from build123d import *

# Parameters (mm, degrees)
SKETCH1_W                    = 7.7
SKETCH1_H                    = 10
BASE_FLANGE1_DEPTH           = 3
EDGE_FLANGE1_STRIP_W         = 13.4732
EDGE_FLANGE1_STRIP_H         = 3
EDGE_FLANGE1_STRIP_CUT_DEPTH = 10
EDGE_FLANGE1_DEPTH           = 10
TAB1_START                   = -3
TAB1_OUTLINE_W               = 23
TAB1_OUTLINE_H               = 10
TAB1_DEPTH                   = 3
FILLET1_R                    = 0.6
FILLET2_R                    = 2
SKETCH15_R                   = 1.75
CUT_EXTRUDE1_DEPTH           = 22.318771072
EDGE_FLANGE2_START           = 2
EDGE_FLANGE2_DEPTH           = 10
EDGE_FLANGE2_2_DEPTH         = 10
CUT_EXTRUDE2_DEPTH           = 31.724582991
FILLET3_R                    = 2


# Read off the part's stored shape, not the designer's step: Tab1, Edge-Flange2
# Sheet-metal steps are written as plain solids
with BuildPart() as part:
    # Sketch1 → Base-Flange1 (new body)
    with BuildSketch(Plane(origin=(0, 0, 0), x_dir=(1, 0, 0), z_dir=(0, 1, 0))):
        with Locations((3.85, 0)):
            Rectangle(SKETCH1_W, SKETCH1_H)
    extrude(amount=-BASE_FLANGE1_DEPTH)

    # Edge-Flange1 strip (across the edge) → Edge-Flange1 strip cut (cut)
    with BuildSketch(Plane(origin=(7.7, 0, 5), x_dir=(-1, 0, 0), z_dir=(0, 0, -1))):
        with Locations((-6, -1.5)):
            Rectangle(EDGE_FLANGE1_STRIP_W, EDGE_FLANGE1_STRIP_H)
    extrude(amount=EDGE_FLANGE1_STRIP_CUT_DEPTH, mode=Mode.SUBTRACT)

    # Edge-Flange1 section (across the edge) → Edge-Flange1 (add)
    with BuildSketch(Plane(origin=(7.7, 0, 5), x_dir=(-1, 0, 0), z_dir=(0, 0, -1))):
        with BuildLine():
            Line((-3, 0.7366), (-3, 2))
            Line((-3, 2), (0, 2))
            Line((0, 2), (0, 0.7366))
            ThreePointArc((0, 0.7366), (0.215745145, 0.215745145), (0.7366, 0))
            Line((0.7366, 0), (0.7366, -3))
            ThreePointArc((0.7366, -3), (-1.905575199, -1.905575199), (-3, 0.7366))
        make_face()
    extrude(amount=EDGE_FLANGE1_DEPTH)

    # Tab1 outline → Tab1 (add)
    with BuildSketch(Plane(origin=(10.7, 0, 0), x_dir=(0, 0, -1), z_dir=(1, 0, 0)).offset(TAB1_START)):
        with Locations((2.5, 7)):
            Rectangle(TAB1_OUTLINE_W, TAB1_OUTLINE_H)
    extrude(amount=TAB1_DEPTH)

    # Fillet1
    fillet1_edges = [part.edges().sort_by_distance(p)[0] for p in [
        (9.2, 2, 5),
        (9.2, 2, -5),
    ]]
    fillet(fillet1_edges, radius=FILLET1_R)

    # Fillet2
    fillet2_edges = [part.edges().sort_by_distance(p)[0] for p in [
        (9.2, 12, -14),
        (9.2, 2, -14),
    ]]
    fillet(fillet2_edges, radius=FILLET2_R)

    # Sketch15 → Cut-Extrude1 (cut, through all)
    with BuildSketch(Plane(origin=(10.7, 0, 0), x_dir=(0, 0, -1), z_dir=(1, 0, 0))):
        with Locations(Location((9, 7, 0), (0, 0, 90))):
            Circle(SKETCH15_R)
    extrude(amount=-CUT_EXTRUDE1_DEPTH, mode=Mode.SUBTRACT)

    # Edge-Flange2 outline → Edge-Flange2 (cut)
    with BuildSketch(Plane(origin=(0, 0, 0), x_dir=(1, 0, 0), z_dir=(0, 1, 0)).offset(EDGE_FLANGE2_START)):
        with BuildLine():
            Line((10.7, -9), (10.7, -8.926677222))
            ThreePointArc((10.7, -8.926677222), (8.545704021, -7.630867001), (7.7, -5.2634))
            Line((7.7, -5.2634), (7.7, -9))
            Line((7.7, -9), (10.7, -9))
        make_face()
    extrude(amount=EDGE_FLANGE2_DEPTH, mode=Mode.SUBTRACT)

    # Edge-Flange2 2 outline → Edge-Flange2 2 (add)
    with BuildSketch(Plane(origin=(0, 0, 0), x_dir=(1, 0, 0), z_dir=(0, 1, 0)).offset(EDGE_FLANGE2_START)):
        with BuildLine():
            ThreePointArc((10.7, -8.926677222), (11.06647982, -8.981624121), (11.4366, -9))
            Line((11.4366, -9), (20, -9))
            Line((20, -9), (20, -6))
            Line((20, -6), (11.4366, -6))
            ThreePointArc((11.4366, -6), (10.915745145, -5.784254855), (10.7, -5.2634))
            Line((10.7, -5.2634), (10.7, -8.926677222))
        make_face()
    extrude(amount=EDGE_FLANGE2_2_DEPTH)

    # Sketch23 → Cut-Extrude2 (cut, through all)
    with BuildSketch(Plane(origin=(0, 0, 6), x_dir=(-1, 0, 0), z_dir=(0, 0, -1))):
        with BuildLine():
            Line((-15.75, 8.65), (-14.25, 8.65))
            ThreePointArc((-14.25, 8.65), (-12.6, 7), (-14.25, 5.35))
            Line((-14.25, 5.35), (-15.75, 5.35))
            ThreePointArc((-15.75, 5.35), (-17.4, 7), (-15.75, 8.65))
        make_face()
    extrude(amount=-CUT_EXTRUDE2_DEPTH, mode=Mode.SUBTRACT)

    # Fillet3
    fillet3_edges = [part.edges().sort_by_distance(p)[0] for p in [
        (20, 12, 7.5),
        (20, 2, 7.5),
    ]]
    fillet(fillet3_edges, radius=FILLET3_R)

    # Mirror1: part across plane


with BuildPart() as part_1:
    add(part.part)
    add(part.part.mirror(Plane(origin=(0, -3, -5), x_dir=(0, 0, 1), z_dir=(-1, 0, 0))))


solid = part_1.part
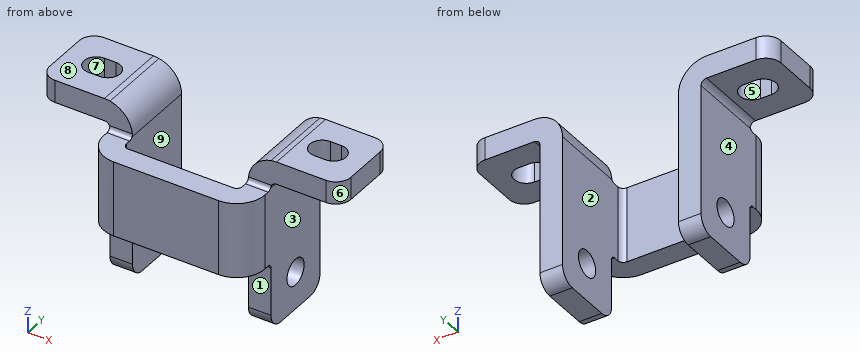
Could you check a few things on this model? Use its own coordinates, in mm. Face numbers are marked on the shaded views. A direction names the side the tool comes from. Coordinates: 2 decimals unless noted, no trailing zeros. Loops run counter-clockwise (first coordinate to the right, second up) from the corner with the lowest first, then second, coordinate; pieces in that order, holes last. Notation, with made-up numbers: (11.5, -35) -> (30.5, -35) arc R19 cw to (30.5, -19) -> close; hole circle Ø7 at (33, -24.5). An arc over 180 degrees is marked (long way). Answer in a Markdown table with one row per item.
(1) Thinking about a two-plate mould opening in X: for the marked faces 6, 7, 8 and 9, which applies, released by +X, released by -X, zero draft, split by the parting line, or undercut?
Results found:
| item | result |
|---|---|
| face 6 | released by +X |
| face 7 | undercut |
| face 8 | zero draft |
| face 9 | undercut |
(2) For the marked faces 1, 2, 3, 4 and 5, which set-ups out of +Z, -Z, +X, -X, +Y, -Y let a thin tool reach every point of the face, with its end or its side?
Results found:
| item | result |
|---|---|
| face 1 | -Z, +X, -X, -Y |
| face 2 | +Z, -Z, +Y |
| face 3 | -Z, +X, +Y, -Y |
| face 4 | -Z, -X, +Y, -Y |
| face 5 | +Z, -Z |
(3) Imagine slicing it at B-B (z = -9). List the corners of the cut face in (x, y) for me.
Results found:
| item | result |
|---|---|
| outline | (-10.7, 2) -> (-7.7, 2) -> (-7.7, 5.25) -> (-10.7, 5.25) -> close; (-10.7, 8.75) -> (-7.7, 8.75) -> (-7.7, 12) -> (-10.7, 12) -> close; (7.7, 2) -> (10.7, 2) -> (10.7, 5.25) -> (7.7, 5.25) -> close; (7.7, 8.75) -> (10.7, 8.75) -> (10.7, 12) -> (7.7, 12) -> close |
(4) Imagine slicing it at D-D (x = 9). List the corners of the cut face in (y, z) for me.
Results found:
| item | result |
|---|---|
| outline | (-2.4, -5) -> (1.4, -5) arc R0.6 cw to (2, -5.6) -> (2, -12) arc R2 ccw to (4, -14) -> (10, -14) arc R2 ccw to (12, -12) -> (12, 8.1) -> (2, 8.1) -> (2, 5.6) arc R0.6 cw to (1.4, 5) -> (-2.4, 5) -> close; hole circle Ø3.5 at (7, -9) |
(5) If I drill on probe 1 along X at (y, z) = (10.25, -9.5); probe 2 along Z at (x, y) = (-8.6, 7); probe 3 along X at (y, z) = (10.5, 7), over which ranges is the centre line in solid material (lowest first)?
Results found:
| item | result |
|---|---|
| probe 1 | x = -10.7 to -7.7, 7.7 to 10.7 |
| probe 2 | z = -14 to -10.75, -7.25 to 7.7 |
| probe 3 | x = -19.94 to -8.13, 8.13 to 19.94 |
(6) Will these pins go through, and if not, where does the flat tip stop? pin 1 Ø0.9 at (x, z) = (9, -10) entering from -Y; pin 2 Ø2 at (y, z) = (1, 2.5) entering from +X; pin 3 Ø5 at (y, z) = (0, 2) entering from -X; pin 4 Ø1 at (x, z) = (-11.5, -11) entering from -Y.
Results found:
| item | result |
|---|---|
| pin 1 | stops at y = 2 |
| pin 2 | stops at x = 10.7 |
| pin 3 | stops at x = -10.7 |
| pin 4 | passes through |
(7) Imagine slicing it at A-A (y = 7). Give the number of separate pieces and of enclosed holes in the cut face, plus the area to 3 significant figures.
Results found:
| item | result |
|---|---|
| separate pieces | 6 |
| enclosed holes | 0 |
| area | 138 mm^2 |
(8) Imagine slicing it at C-C (z = -4.25). List the corners of the cut face in (x, y) for me, plus the area to 3 significant figures.
Results found:
| item | result |
|---|---|
| outline | (-10.7, 0.74) arc R3.74 ccw to (-6.96, -3) -> (6.96, -3) arc R3.74 ccw to (10.7, 0.74) -> (10.7, 12) -> (7.7, 12) -> (7.7, 0.74) arc R0.74 cw to (6.96, 0) -> (-6.96, 0) arc R0.74 cw to (-7.7, 0.74) -> (-7.7, 12) -> (-10.7, 12) -> close |
| area | 130 mm^2 |
